For this review, take the finished solid that the model builds, in its own axes (mm). Coordinates: 2 decimals unless noted, no trailing zeros. Write each loop counter-clockwise with the first axis right and the second up, starting at its lowest first coordinate (ties: lowest second). Pieces come first, ordered by that corner, then holes. Notation, with made-up numbers: M 32,0 L 57,0 A21 cw 57,39 Z; hole C -17,79.25 d3. An arc over 180 degrees is marked long. Return JSON: item names as keys, results as strings.
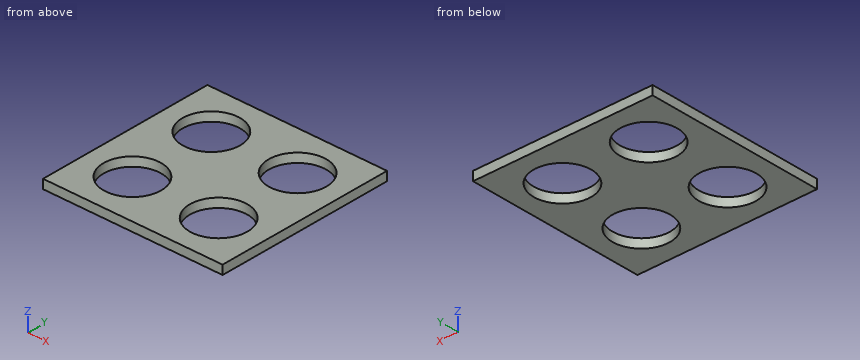
Autodesk Inventor part; units mm, degrees
ref_plane "YZ Plane" through (0, 0, 0) normal (1, 0, 0) x (0, 1, 0)
ref_plane "XZ Plane" through (0, 0, 0) normal (0, 1, 0) x (-1, 0, 0)
ref_plane "XY Plane" through (0, 0, 0) normal (0, 0, 1) x (1, 0, 0)
sketch "Sketch1" plane through (0, 0, 0) normal (0, 0, 1) x (1, 0, 0)
  line L0 (0, 0) -> (100, 0)
  line L1 (100, 0) -> (100, 100)
  line L2 (100, 100) -> (0, 100)
  line L3 (0, 100) -> (0, 0)
  dimension "d0" = 100
  dimension "d1" = 100
extrude "Extrusion1" add sketch "Sketch1" along normal blind 5
sketch "Sketch2" plane through (0, 0, 5) normal (0, 0, 1) x (1, 0, 0)
  line L0 (100, 100) -> (0, 100) construction
  line L1 (0, 0) -> (100, 0) construction
  line L2 (100, 0) -> (100, 100) construction
  line L3 (0, 100) -> (0, 0) construction
  circle A0 centre (26, 74) radius 16
  circle A1 centre (74, 26) radius 16
  circle A2 centre (74, 74) radius 16
  circle A3 centre (26, 26) radius 16
  dimension "d4" = 32
  dimension "d5" = 32
  dimension "d6" = 32
  dimension "d7" = 32
  dimension "d15" = 26
  dimension "d16" = 26
  dimension "d17" = 26
  dimension "d18" = 26
  dimension "d19" = 26
  dimension "d20" = 26
  dimension "d21" = 26
  dimension "d22" = 26
  dimension "d23" = 48
  dimension "d24" = 48
  dimension "d25" = 48
  dimension "d26" = 48
extrude "Extrusion3" cut sketch "Sketch2" against normal blind 5
equation "\"d0\" = tankw"
equation "\"d1\" = sensorsupportl"
equation "\"d2\" = pvct"
equation "\"d4\" = diahcl"
equation "\"d5\" = diaph"
equation "\"d6\" = diacucl"
equation "\"d7\" = diaetape"
equation "\"d15\" = 0.5 * diahcl + 2 * pvct"
equation "\"d16\" = 0.5 * diahcl + 2 * pvct"
equation "\"d17\" = 0.5 * diacucl + 2 * pvct"
equation "\"d18\" = 0.5 * diacucl + 2 * pvct"
equation "\"d19\" = 0.5 * diaph + 2 * pvct"
equation "\"d20\" = 0.5 * diaph + 2 * pvct"
equation "\"d21\" = 0.5 * diaetape + 2 * pvct"
equation "\"d22\" = 0.5 * diaetape + 2 * pvct"
equation "\"d29\" = pvct"
equation "\"lcsd\" = 19.05"
equation "\"lcwd1\" = 25"
equation "\"lcwd2\" = 34"
equation "\"lch1\" = 39"
equation "\"lcwd3\" = 43"
equation "\"dia1\" = 6"
equation "\"td\" = 18"
equation "\"bhh\" = 6"
equation "\"sw\" = 25"
equation "\"sh\" = 31"
equation "\"spacert\" = 2"
equation "\"pvct\" = 5"
equation "\"tankw\" = 100"
equation "\"tankl\" = 379"
equation "\"dia3\" = 8"
equation "\"dia4\" = 11"
equation "\"play\" = 9"
equation "\"holeh\" = 26"
equation "\"surroundt\" = 5"
equation "\"slack\" = 0.5"
equation "\"play2\" = 3"
equation "\"diaoverflow\" = 25"
equation "\"diacucl\" = 32"
equation "\"diawater\" = 25"
equation "\"diaph\" = 32"
equation "\"diaair\" = 32"
equation "\"diasurroundhole\" = 42"
equation "\"sensorsupportl\" = 100"
equation "\"diagrate\" = 12"
equation "\"gratespacing\" = 12.02082"
equation "\"sidedist\" = 13.9375"
equation "\"bottomdist\" = 9.6355"
equation "\"diahcl\" = 32"
equation "\"bracketwtop\" = 6"
equation "\"bracketwbottom\" = 6"
equation "\"nett\" = 1"
equation "\"nethole\" = 16"
equation "\"netside\" = 3.5"
equation "\"nettop\" = 7"
equation "\"netholespacing\" = 2"
equation "\"diaetape\" = 32"
properties part number "tank_front" material "PVC-Piping"
1. Wall thickness on L1, parallel to Y at x = 74, z = 3.7; L2, parallel to X at y = 87.5, z = 2.1; L3, parallel to X at y = 80, z = 1.9: over which ranges is each line inside the solid? List them lowest first. Write a range as from..to.
Checks:
{"L1": "0..10, 42..58, 90..100", "L2": "0..17.41, 34.59..65.41, 82.59..100", "L3": "0..11.17, 40.83..59.17, 88.83..100"}
2. We need section C-C (z = 0.8). State the section outline as (x, y) points.
Checks:
{"outline": "M 0,0 L 100,0 L 100,100 L 0,100 Z; hole C 26,26 d32; hole C 26,74 d32; hole C 74,26 d32; hole C 74,74 d32"}
3. We need section A-A (y = 20.5). State the section outline as (x, z) points, plus the area to 4 significant figures.
Checks:
{"outline": "M 0,0 L 10.98,0 L 10.98,5 L 0,5 Z; M 41.02,0 L 58.98,0 L 58.98,5 L 41.02,5 Z; M 89.02,0 L 100,0 L 100,5 L 89.02,5 Z", "area": "199.5 mm2"}
4. We need section B-B (x = 26). State the section outline as (y, z) points, plus the area to 3 significant figures.
Checks:
{"outline": "M 0,0 L 10,0 L 10,5 L 0,5 Z; M 42,0 L 58,0 L 58,5 L 42,5 Z; M 90,0 L 100,0 L 100,5 L 90,5 Z", "area": "180 mm2"}
